Read the model definition and answer for the solid it produces. Units are mm, in the model's axes. A direction names the side the tool comes from. Coordinates: 2 decimals unless noted, no trailing zeros. Use one line per item in the form item = value. Start each with the question number.
1) Which of the six approach directions +Z, -Z, +X, -X, +Y, -Y give full straight-line access (tool end or side, diameter ignored) to faces 1 (the face through (43.047, -163.173, -21.424)), 2 (the face through (-74.926, 159.655, -35.453)), 3 (the face through (30.81, 52.716, -11.706))?
2) Each of these flat-tipped pins is pushed along its axis until it touches: P1, Ø8, axis at y = -94.5, z = -56.5, coming from the -X side; P2, Ø8, axis at y = 75, z = -77.5, coming from the +X side; P3, Ø5, axis at x = -61, y = -25, coming from the -Z side. Where does it stop, or does it pass through?
3) Consider line 1 (X direction, y = 70.5, z = 165.5); line 2 (Y direction, x = 0.5, z = 0); line 3 (X direction, y = 56, z = -57). Determine where each line is inside the solid, lowest interval first.
4) The mould has two halves that part along Z. Classify faces 4 (the face through (26.5, -50, 23)), 5 (the face through (-42.924, 100, -130.417)): released by +Z, released by -Z, zero draft, split by the parting line, or undercut.
from build123d import *


with BuildPart() as part:
    # Sketch1 → Revolve2 (revolve)
    with BuildSketch(Plane.XY, mode=Mode.PRIVATE) as revolve2_sk:
        Polygon((-35, 20), (-35, 54), (-26.5, 54), (-26.5, 108.596183719), (-80, 133.54364343), (-80, 163.54364343), (-69.991642542, 163.54364343), (-61.241642543, 180), (-51.241642542, 180), (-42.500000003, 163.54364343), (-32.500000001, 163.54364343), (-23.750000002, 180), (-13.75, 180), (-5.000000001, 163.54364343), (5.000000001, 163.54364343), (13.75, 180), (23.750000002, 180), (32.500000001, 163.54364343), (42.500000003, 163.54364343), (51.241642542, 180), (61.241642543, 180), (69.991642542, 163.54364343), (80, 163.54364343), (80, 133.54364343), (26.5, 108.596183719), (26.5, 54), (35, 54), (35, 20), align=None)
    revolve(revolve2_sk.sketch.rotate(Axis((-35, 0, 0), (1, 0, 0)), 90), axis=Axis((-35, 0, 0), (1, 0, 0)))


solid = part.part
Found:
q1.face_1 = none
q1.face_2 = -X
q1.face_3 = +X
q2.P1 = -38.31
q2.P2 = 33.47
q2.P3 = -178.59
q3.line_1 = -61.3 to -51.18, -23.81 to -13.69, 13.69 to 23.81, 51.18 to 61.3
q3.line_2 = -163.54 to -20, 20 to 163.54
q3.line_3 = -26.5 to 26.5
q4.face_4 = undercut
q4.face_5 = split by the parting line
